The drawing under review shows one solid part. Ordinate dimensions are in mm from its lowest x, y, z. A direction names the side the tool comes from. Coordinates: 2 decimals unless noted, no trailing zeros. Write each loop counter-clockwise with the first axis right and the second up, starting at its lowest first coordinate (ties: lowest second). Pieces come first, ordered by that corner, then holes. Notation, with made-up numbers: M 36,44 L 50,44 A6 ccw 50,50 Z; hole C 17,-11.5 d4. An arc over 180 degrees is marked long. Write item = value, one per line.
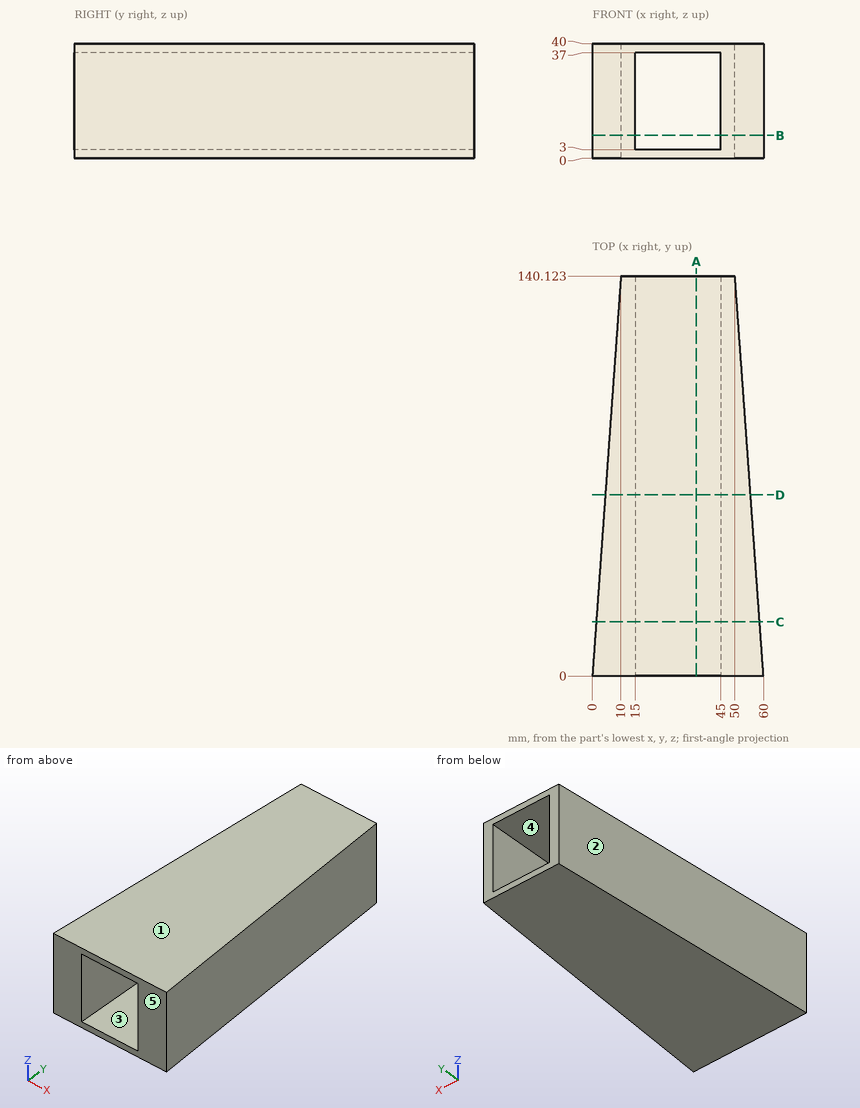
Q1. Machinability: for the marked faces 4 and 5, which of the approach directions +Z, -Z, +X, -X, +Y, -Y give a long, thin tool a straight path to every point of the face, cutting with its end or side? Answer none if there is none.
Check result:
face_4 = +Y, -Y
face_5 = +Z, -Z, +X, -X, -Y
Q2. Wall thickness on line 1 (Z direction, x = 43, y = 55.5); line 2 (X direction, y = 71, z = 9); line 3 (X direction, y = 24.5, z = 36): over which ranges is each line inside the solid? List them lowest first.
Check result:
line_1 = 0 to 3, 37 to 40
line_2 = 5.07 to 15, 45 to 54.93
line_3 = 1.75 to 15, 45 to 58.25
Q3. The part is to be moulded in two halves that separate along Z. For the marked faces 1, 2 and 3, say which applies: +Z half, -Z half, draft (parallel to the pull), parting line (faces both ways), or undercut.
Check result:
face_1 = +Z half
face_2 = draft
face_3 = undercut
Q4. Consider section C-C, the plane y = 19. State the section outline as (x, z) points.
Check result:
outline = M 1.36,0 L 58.64,0 L 58.64,40 L 1.36,40 Z; hole M 15,3 L 45,3 L 45,37 L 15,37 Z
Q5. For P1, Ø5, axis at y = 67, z = 9, coming from the +X side; P2, Ø10, axis at y = 105, z = 14, coming from the -X side; P3, Ø2, axis at y = 53.5, z = 4.5, coming from the -X side; P4, Ø4, axis at x = 18.5, z = 33.5, coming from the +Y side, all flat-tipped, find the tip position at first contact; note any pin that passes through.
Check result:
P1 = 55.4
P2 = 7.14
P3 = 3.75
P4 = through
Q6. Consider section A-A, the plane x = 36.5. State the section outline as (y, z) points.
Check result:
outline = M 0,0 L 140.12,0 L 140.12,3 L 0,3 Z; M 0,37 L 140.12,37 L 140.12,40 L 0,40 Z
Q7. Consider section D-D, the plane y = 63.5. State the section outline as (x, z) points.
Check result:
outline = M 4.53,0 L 55.47,0 L 55.47,40 L 4.53,40 Z; hole M 15,3 L 45,3 L 45,37 L 15,37 Z
Q8. Consider section B-B, the plane z = 8. State the section outline as (x, y) points.
Check result:
outline = M 0,0 L 15,0 L 15,140.12 L 10,140.12 Z; M 45,0 L 60,0 L 50,140.12 L 45,140.12 Z
